Part model, mm, in its own coordinate system. Give positions to 0.01 mm unless a question says otherwise; leave off trailing zeros. Write each loop counter-clockwise with the first axis right and the second up, starting at its lowest first coordinate (ties: lowest second). Pieces come first, ordered by that corner, then holes.
from build123d import *

# Parameters (mm, degrees)
SKETCH1_W           = 330
SKETCH1_H           = 50
BOSS_EXTRUDE1_DEPTH = 35
SKETCH2_R           = 12.7
CUT_EXTRUDE1_DEPTH  = 70
SKETCH3_R           = 5
CUT_EXTRUDE2_DEPTH  = 70
SKETCH4_R           = 5
CUT_EXTRUDE3_DEPTH  = 43


with BuildPart() as part:
    # Sketch1 → Boss-Extrude1 (new body)
    with BuildSketch(Plane(origin=(0, 0, 0), x_dir=(1, 0, 0), z_dir=(0, 1, 0))):
        Rectangle(SKETCH1_W, SKETCH1_H)
    extrude(amount=BOSS_EXTRUDE1_DEPTH)

    # Sketch2 → Cut-Extrude1 (cut)
    with BuildSketch(Plane(origin=(0, 35, 0), x_dir=(1, 0, 0), z_dir=(0, 1, 0))):
        with Locations((-100, 0)):
            Circle(SKETCH2_R)
        with Locations((100, 0)):
            Circle(SKETCH2_R)
    extrude(amount=-CUT_EXTRUDE1_DEPTH, mode=Mode.SUBTRACT)

    # Sketch3 → Cut-Extrude2 (cut)
    with BuildSketch(Plane.XY.offset(25)):
        with Locations((-100, 17.5)):
            Circle(SKETCH3_R)
        with Locations((100, 17.5)):
            Circle(SKETCH3_R)
    extrude(amount=-CUT_EXTRUDE2_DEPTH, mode=Mode.SUBTRACT)

    # Sketch4 → Cut-Extrude3 (cut)
    with BuildSketch(Plane(origin=(0, 35, 0), x_dir=(1, 0, 0), z_dir=(0, 1, 0))):
        Circle(SKETCH4_R)
    extrude(amount=-CUT_EXTRUDE3_DEPTH, mode=Mode.SUBTRACT)


solid = part.part
1) Mould opens along X. For faces 1 (the flat face through (-2, 17, -25)), 2 (the cylindrical face through (112.114, 17.745, -3.815)), 3 (the flat face through (165, 17, 0)) say: +X half, -X half, draft (parallel to the pull), parting line (faces both ways), or undercut.
Check result:
face 1: draft
face 2: undercut
face 3: +X half
2) Saw through at C-C (x = 0). Write the cut outline in (y, z).
Check result:
outline: (0, -25) - (35, -25) - (35, -5) - (0, -5) - close; (0, 5) - (35, 5) - (35, 25) - (0, 25) - close
3) Saw through at A-A (y = 17.5). Write the cut outline in (x, z), and give its area (3 significant figures).
Check result:
outline: (-165, -25) - (-105, -25) - (-105, -11.67) arc R12.7 cw to (-105, 11.67) - (-105, 25) - (-165, 25) - close; (-95, -25) - (95, -25) - (95, -11.67) arc R12.7 cw to (95, 11.67) - (95, 25) - (-95, 25) - (-95, 11.67) arc R12.7 cw to (-95, -11.67) - close; (105, -25) - (165, -25) - (165, 25) - (105, 25) - (105, 11.67) arc R12.7 cw to (105, -11.67) - close; hole circle Ø10 at (0, 0)
area: 14,900 mm2
4) Saw through at B-B (z = 0). Write the cut outline in (x, y).
Check result:
outline: (-165, 0) - (-112.7, 0) - (-112.7, 35) - (-165, 35) - close; (-87.3, 0) - (-5, 0) - (-5, 35) - (-87.3, 35) - close; (5, 0) - (87.3, 0) - (87.3, 35) - (5, 35) - close; (112.7, 0) - (165, 0) - (165, 35) - (112.7, 35) - close
5) Saw through at D-D (x = 100). Write the cut outline in (y, z).
Check result:
outline: (0, -25) - (12.5, -25) - (12.5, -12.7) - (0, -12.7) - close; (0, 12.7) - (12.5, 12.7) - (12.5, 25) - (0, 25) - close; (22.5, -25) - (35, -25) - (35, -12.7) - (22.5, -12.7) - close; (22.5, 12.7) - (35, 12.7) - (35, 25) - (22.5, 25) - close
6) Drill centre lines: L1, parallel to X at y = 19, z = 0; L2, parallel to X at y = 17.5, z = 16; L3, parallel to X at y = 20.5, z = 14.5. Where is each one in solid material? Low to high.
Check result:
L1: x = -165 to -112.7, -87.3 to -5, 5 to 87.3, 112.7 to 165
L2: x = -165 to -105, -95 to 95, 105 to 165
L3: x = -165 to -104, -96 to 96, 104 to 165
